Autodesk Inventor part; units mm, degrees
ref_plane "YZ Plane" through (0, 0, 0) normal (1, 0, 0) x (0, 1, 0)
ref_plane "XZ Plane" through (0, 0, 0) normal (0, 1, 0) x (-1, 0, 0)
ref_plane "XY Plane" through (0, 0, 0) normal (0, 0, 1) x (1, 0, 0)
sketch "Sketch1" plane through (0, 0, 0) normal (0, 1, 0) x (-1, 0, 0)
  line L0 (0, 0) -> (200, 0)
  line L1 (200, 0) -> (200, -150)
  line L2 (200, -150) -> (0, -150)
  line L3 (0, -150) -> (0, 0)
  dimension "d0" = 200
  dimension "d1" = 150
extrude "Extrusion1" add sketch "Sketch1" along normal blind 10
sketch "Sketch2" plane through (0, 0, 0) normal (0, -1, 0) x (1, 0, 0)
  line L0 (-199.8, -85) -> (-186.3697, -85) construction
  line L1 (-187.7125, -90.8572) -> (-200, -85.1274)
  line L2 (-200, -85.1274) -> (-200, -64.8726)
  line L3 (-200, -64.8726) -> (-187.7125, -59.1428)
  arc A0 (-186.0054, -60.2304) -> (-187.7125, -59.1428) centre (-187.2054, -60.2304) ccw
  line L4 (-186.0054, -60.2304) -> (-186.0054, -75)
  line L5 (-186.0054, -75) -> (-186.0054, -89.7696)
  arc A1 (-187.7125, -90.8572) -> (-186.0054, -89.7696) centre (-187.2054, -89.7696) ccw
  line L6 (-200, -150) -> (-200, 0)
  point P0 (0, 0)
  point P1 (-186.2054, -91.3393)
  point P2 (-200, -75)
  point P3 (-200, -75)
  dimension "d4" = 15
extrude "Extrusion2" cut sketch "Sketch2" against normal blind 5.2
sketch "Sketch3" plane through (0, 0, 0) normal (0, -1, 0) x (1, 0, 0)
  line L0 (-110, -149.8) -> (-110, -163.2303) construction
  line L1 (-100, -163.1946) -> (-114.7696, -163.1946)
  arc A0 (-115.4946, -162.0565) -> (-114.7696, -163.1946) centre (-114.7696, -162.3946) ccw
  line L2 (-115.4946, -162.0565) -> (-109.8726, -150)
  line L3 (-109.8726, -150) -> (-90.1274, -150)
  line L4 (-90.1274, -150) -> (-84.5054, -162.0565)
  arc A1 (-85.2304, -163.1946) -> (-84.5054, -162.0565) centre (-85.2304, -162.3946) ccw
  line L5 (-85.2304, -163.1946) -> (-100, -163.1946)
  line L6 (0, -150) -> (-200, -150)
  point P0 (0, 0)
  point P1 (-100, -150)
  point P2 (-100, -150)
  point P3 (-100, -150)
extrude "Extrusion3" add sketch "Sketch3" against normal blind 4.8
sketch "Sketch4" plane through (0, 10, 0) normal (0, 1, 0) x (1, 0, 0)
  line L0 (-200, 85.1274) -> (-200, 64.8726)
  line L1 (0, 0) -> (0, 150)
  line L2 (0, 75) -> (-75, 75)
  circle A0 centre (-200, 75) radius 2.6
  circle A1 centre (-75, 75) radius 2.6
  dimension "d12" = 75
  dimension "d13" = 5.2
  dimension "d14" = 5.2
extrude "Extrusion4" cut sketch "Sketch4" against normal blind 5.2
sketch "Sketch5" plane through (0, 10, 0) normal (0, 1, 0) x (1, 0, 0)
  line L0 (-200, 0) -> (0, 0)
  line L1 (0, 150) -> (-50, 150)
  line L2 (-50, 150) -> (-50, 0)
  line L3 (-50, 0) -> (0, 0)
  line L4 (0, 0) -> (0, 150)
  line L5 (-200, 0) -> (0, 0)
  line L6 (0, 0) -> (0, 50)
  line L7 (0, 50) -> (-200, 50)
  line L8 (-200, 50) -> (-200, 0)
  line L9 (-200, 150) -> (-130, 150)
  line L10 (-130, 150) -> (-130, 100)
  line L11 (-130, 100) -> (-200, 100)
  line L12 (-200, 100) -> (-200, 150)
  point P0 (-50, 50)
  dimension "d17" = 50
  dimension "d18" = 50
  dimension "d19" = 70
  dimension "d20" = 50
extrude "Extrusion5" cut sketch "Sketch5" against normal blind 15
fillet "Fillet1" radius 10 6 edges at (-50, 5, -150) (-130, 5, -150) (-200, 5, -100) (-130, 5, -100) (-200, 5, -50) (-50, 5, -50)
properties part number "Area nh"
For this review, take the finished solid that the model builds, in its own axes (mm). A direction names the side the tool comes from. Coordinates: 2 decimals unless noted, no trailing zeros. Write each loop counter-clockwise with the first axis right and the second up, starting at its lowest first coordinate (ties: lowest second). Pieces come first, ordered by that corner, then holes. Notation, with made-up numbers: (40, 42) - (75, 42) arc R26 ccw to (75, 76) - close; hole circle Ø7 at (64, -13). An arc over 180 degrees is marked (long way). Answer in a Markdown table with one row per item. Add a question column.
Q1. For P1, Ø5, axis at x = -95.5, z = -124.5, coming from the -Y side; P2, Ø4, axis at x = -75, z = -75, coming from the +Y side; P3, Ø5.5, axis at y = 1.5, z = -75, coming from the -X side; P4, Ø2, axis at x = -156, y = 6, coming from the -Z side, all flat-tipped, find the tip position at first contact; note any pin that passes through.
Q2. We need section D-D, the plane z = -88. State the section outline as (x, y) points, and give its area (3 significant figures).
Q3. For probe 1 along Z at (x, y) = (-75, 7.9); probe 2 along X at (y, z) = (7.6, -75); probe 3 along Z at (x, y) = (-84, 4.75), list the stretches that pass through material, from the lowest coordinate up.
Q4. We need section A-A, the plane y = 7.5. State the section outline as (x, z) points.
Q5. We need section B-B, the plane z = -75. State the section outline as (x, y) points.
Q6. Draft analysis for pull direction X (two halves, no side actions). For faces 1 (the cylindrical face through (-76.916, 7.436, -76.757)), 2 (the flat face through (-165, 5, -100)), 3 (the cylindrical face through (-52.85, 4.93, -53.01)), 4 (the flat face through (-200, 6, -85)), state which applies: +X half, -X half, draft (parallel to the pull), parting line (faces both ways), or undercut.
Q7. We need section C-C, the plane x = -75. State the section outline as (y, z) points.
Q8. Tool access review of faces 5 (the flat face through (-87.356, 2.366, -155.944)), 6 (the flat face through (-193.942, 2.564, -62.048)), 7 (the flat face through (-130, 5, -125)), 8 (the flat face through (-112.72, 2.37, -156.11)): name each direction out of +Z, -Z, +X, -X, +Y, -Y from which nothing blocks a thin tool from reaching the whole face with its end or side.
Answer list:
| question | item | result |
|---|---|---|
| 1 | P1 | stops at y = 0 |
| 1 | P2 | stops at y = 4.8 |
| 1 | P3 | stops at x = -186.01 |
| 1 | P4 | stops at z = -100 |
| 2 | outline | (-200, 0) - (-193.84, 0) - (-193.84, 5.2) - (-186.01, 5.2) - (-186.01, 0) - (-50, 0) - (-50, 10) - (-200, 10) - close |
| 2 | area | 1,460 mm2 |
| 3 | probe 1 | z = -150 to -77.6, -72.4 to -50 |
| 3 | probe 2 | x = -197.4 to -77.6, -72.4 to -50 |
| 3 | probe 3 | z = -150 to -50 |
| 4 | outline | (-200, -90) arc R10 ccw to (-190, -100) - (-140, -100) arc R10 cw to (-130, -110) - (-130, -140) arc R10 ccw to (-120, -150) - (-60, -150) arc R10 ccw to (-50, -140) - (-50, -60) arc R10 ccw to (-60, -50) - (-190, -50) arc R10 ccw to (-200, -60) - (-200, -72.4) arc R2.6 cw to (-200, -77.6) - close; hole circle Ø5.2 at (-75, -75) |
| 5 | outline | (-197.4, 5.2) - (-186.01, 5.2) - (-186.01, 0) - (-50, 0) - (-50, 10) - (-72.4, 10) - (-72.4, 4.8) - (-77.6, 4.8) - (-77.6, 10) - (-197.4, 10) - close |
| 6 | face 1 | undercut |
| 6 | face 2 | draft |
| 6 | face 3 | +X half |
| 6 | face 4 | -X half |
| 7 | outline | (0, -150) - (10, -150) - (10, -77.6) - (4.8, -77.6) - (4.8, -72.4) - (10, -72.4) - (10, -50) - (0, -50) - close |
| 8 | face 5 | +X, +Y, -Y |
| 8 | face 6 | -Y |
| 8 | face 7 | -Z, -X, +Y, -Y |
| 8 | face 8 | -X, +Y, -Y |
